Geometry check sheet. Reference: the model listing, model coordinates, mm. A direction names the side the tool comes from. Round coordinates to 2 decimals unless told otherwise and drop trailing zeros. Loops run counter-clockwise (first coordinate to the right, second up) from the corner with the lowest first, then second, coordinate; pieces in that order, holes last. Notation, with made-up numbers: M 35,-20 L 85,-20 A12 cw 85,-11 Z; hole C 63.25,41 d8. An arc over 180 degrees is marked long. Write item = value, one per line.
from build123d import *

# Parameters (mm, degrees)
F0_W     = 3
F0_H     = 30
F1_DEPTH = 52.5
F3_DEPTH = 25
F4_R     = 2
F6_DEPTH = 25


# Not quite as in the source:
# - a feature names something its author has since deleted; it is built from what else it names


with BuildPart() as f1:
    # F0 (on Top) → F1 (new body)
    with BuildSketch(Plane.XY):
        Polygon((2, 0), (-1, 0), (-6.1, 0), (-6.1, 30), (-9.1, 30), (-9.1, -2.9952730983), (40, -3), (40, 0), align=None)
        with Locations((0.5, 15)):
            Rectangle(F0_W, F0_H)
    extrude(amount=F1_DEPTH)

    # F2 (on face) → F3 (cut)
    with BuildSketch(Plane(origin=(-9.1, 0, 0), x_dir=(0, -1, 0), z_dir=(-1, 0, 0))):
        with BuildLine():
            Line((-13.5023634508, 37.5), (-13.5023634508, 39.25))
            ThreePointArc((-13.5023634508, 39.25), (-15.2523634508, 37.5), (-13.5023634508, 35.75))
            Line((-13.5023634508, 35.75), (-13.5023634508, 37.5))
        make_face()
        with BuildLine():
            ThreePointArc((-11.7523634508, 37.5), (-12.2649265837, 38.7374368671), (-13.5023634508, 39.25))
            Line((-13.5023634508, 39.25), (-13.5023634508, 37.5))
            Line((-13.5023634508, 37.5), (-13.5023634508, 35.75))
            ThreePointArc((-13.5023634508, 35.75), (-12.2649265837, 36.2625631329), (-11.7523634508, 37.5))
        make_face()
        with BuildLine():
            Line((-13.5023634508, 15), (-13.5023634508, 13.25))
            ThreePointArc((-13.5023634508, 13.25), (-12.2649265837, 13.7625631329), (-11.7523634508, 15))
            ThreePointArc((-11.7523634508, 15), (-12.2649265837, 16.2374368671), (-13.5023634508, 16.75))
            Line((-13.5023634508, 16.75), (-13.5023634508, 15))
        make_face()
        with BuildLine():
            ThreePointArc((-13.5023634508, 16.75), (-15.2523634508, 15), (-13.5023634508, 13.25))
            Line((-13.5023634508, 13.25), (-13.5023634508, 15))
            Line((-13.5023634508, 15), (-13.5023634508, 16.75))
        make_face()
    extrude(amount=-F3_DEPTH, mode=Mode.SUBTRACT)

    # F4
    f4_edges = [f1.edges().sort_by_distance(p)[0] for p in [
        (40, -1.5, 52.5),
        (-9.1, 30, 26.25),
        (-9.1, 13.502363, 52.5),
        (-7.6, 30, 52.5),
    ]]
    fillet(f4_edges, radius=F4_R)

    # F5 (on face) → F6 (cut)
    with BuildSketch(Plane(origin=(-0.000288442, -2.9961491359, 0), x_dir=(0.9999999954, -9.62709e-05, 0), z_dir=(-9.62709e-05, -0.9999999954, 0))):
        with BuildLine():
            Line((15.0002886274, 35), (15.0002886274, 33.25))
            ThreePointArc((15.0002886274, 33.25), (16.2377254944, 33.7625631329), (16.7502886274, 35))
            Line((16.7502886274, 35), (15.0002886274, 35))
        make_face()
        with BuildLine():
            ThreePointArc((15.0002886274, 36.75), (13.2502886274, 35), (15.0002886274, 33.25))
            Line((15.0002886274, 33.25), (15.0002886274, 35))
            Line((15.0002886274, 35), (15.0002886274, 36.75))
        make_face()
        with BuildLine():
            Line((15.0002886274, 36.75), (15.0002886274, 35))
            Line((15.0002886274, 35), (16.7502886274, 35))
            ThreePointArc((16.7502886274, 35), (16.2377254944, 36.2374368671), (15.0002886274, 36.75))
        make_face()
        with BuildLine():
            Line((30.0002886274, 35), (31.7502886274, 35))
            ThreePointArc((31.7502886274, 35), (31.2377254944, 36.2374368671), (30.0002886274, 36.75))
            Line((30.0002886274, 36.75), (30.0002886274, 35))
        make_face()
        with BuildLine():
            Line((28.2502886274, 35), (30.0002886274, 35))
            Line((30.0002886274, 35), (30.0002886274, 36.75))
            ThreePointArc((30.0002886274, 36.75), (28.7628517603, 36.2374368671), (28.2502886274, 35))
        make_face()
        with BuildLine():
            Line((30.0002886274, 33.25), (30.0002886274, 35))
            Line((30.0002886274, 35), (28.2502886274, 35))
            ThreePointArc((28.2502886274, 35), (28.7628517603, 33.7625631329), (30.0002886274, 33.25))
        make_face()
        with BuildLine():
            ThreePointArc((30.0002886274, 33.25), (31.2377254944, 33.7625631329), (31.7502886274, 35))
            Line((31.7502886274, 35), (30.0002886274, 35))
            Line((30.0002886274, 35), (30.0002886274, 33.25))
        make_face()
        with BuildLine():
            Line((30.0002886274, 15), (31.7502886274, 15))
            ThreePointArc((31.7502886274, 15), (31.2377254944, 16.2374368671), (30.0002886274, 16.75))
            Line((30.0002886274, 16.75), (30.0002886274, 15))
        make_face()
        with BuildLine():
            Line((28.2502886274, 15), (30.0002886274, 15))
            Line((30.0002886274, 15), (30.0002886274, 16.75))
            ThreePointArc((30.0002886274, 16.75), (28.7628517603, 16.2374368671), (28.2502886274, 15))
        make_face()
        with BuildLine():
            ThreePointArc((28.2502886274, 15), (28.7628517603, 13.7625631329), (30.0002886274, 13.25))
            Line((30.0002886274, 13.25), (30.0002886274, 15))
            Line((30.0002886274, 15), (28.2502886274, 15))
        make_face()
        with BuildLine():
            Line((30.0002886274, 15), (30.0002886274, 13.25))
            ThreePointArc((30.0002886274, 13.25), (31.2377254944, 13.7625631329), (31.7502886274, 15))
            Line((31.7502886274, 15), (30.0002886274, 15))
        make_face()
        with BuildLine():
            Line((15.0002886274, 15), (15.0002886274, 13.25))
            ThreePointArc((15.0002886274, 13.25), (16.2377254944, 13.7625631329), (16.7502886274, 15))
            Line((16.7502886274, 15), (15.0002886274, 15))
        make_face()
        with BuildLine():
            Line((15.0002886274, 16.75), (15.0002886274, 15))
            Line((15.0002886274, 15), (16.7502886274, 15))
            ThreePointArc((16.7502886274, 15), (16.2377254944, 16.2374368671), (15.0002886274, 16.75))
        make_face()
        with BuildLine():
            ThreePointArc((15.0002886274, 16.75), (13.2502886274, 15), (15.0002886274, 13.25))
            Line((15.0002886274, 13.25), (15.0002886274, 15))
            Line((15.0002886274, 15), (15.0002886274, 16.75))
        make_face()
    extrude(amount=-F6_DEPTH, mode=Mode.SUBTRACT)


solid = f1.part
(1) Material ranges on line 1 along X through (y, z) = (24, 7); line 2 along Y through (x, z) = (1.5, 33); line 3 along Y through (x, z) = (7, 50), recorded low to high. Write a range as from..to.
Result set:
line_1 = -9.1..-6.1, -1..2
line_2 = -3..30
line_3 = -3..0
(2) Depth check by flat-ended pin: pin 1 Ø2 at (x, z) = (3.5, 36.5) entering from +Y; pin 2 Ø4 at (x, z) = (10.5, 15.5) entering from -Y; pin 3 Ø6 at (y, z) = (25, 37) entering from +X; pin 4 Ø1.5 at (x, y) = (2, 18.5) entering from -Z. Enter the tip coordinate at first touch or a pass-through.
Result set:
pin_1 = 0
pin_2 = -3
pin_3 = 2
pin_4 = 0
(3) Release check for a two-part mould opening along X. For faces 1 (the flat face through (1, 9, 0)), 2 (the cylindrical face through (39.4, -1.48, 51.93)), 3 (the flat face through (-4, 0, 26)), 4 (the flat face through (-1, 15, 26)) record: released by +X, released by -X, zero draft, split by the parting line, or undercut.
Result set:
face_1 = zero draft
face_2 = released by +X
face_3 = undercut
face_4 = undercut
(4) Sectioned sample at B-B on z = 24.5. Record the cut outline in (x, y).
Result set:
outline = M -9.1,-3 L 40,-3 L 40,0 L 2,0 L 2,30 L -1,30 L -1,0 L -6.1,0 L -6.1,30 L -7.1,30 A2 ccw -9.1,28 Z
(5) Sectioned sample at A-A on y = 4.5. Record the cut outline in (x, z).
Result set:
outline = M -9.1,0 L -6.1,0 L -6.1,52.5 L -7.1,52.5 A2 ccw -9.1,50.5 Z; M -1,0 L 2,0 L 2,52.5 L -1,52.5 Z
(6) Tool access check on faces 5 (the cylindrical face through (-6.61, 29.4, 51.93)), 6 (the flat face through (40, -2, 25)), 7 (the flat face through (-6.1, 15, 26)), 8 (the flat face through (21, 0, 26)), 9 (the flat face through (0, 30, 26)). Record the directions out of +Z, -Z, +X, -X, +Y, -Y that give a thin tool (end or side, any length) a straight path to the whole face; none if there is none.
Result set:
face_5 = +Z, -X, +Y
face_6 = +Z, -Z, +X, +Y, -Y
face_7 = +Z, -Z, +Y
face_8 = +Z, -Z, +X, +Y
face_9 = +Z, -Z, +X, -X, +Y
(7) Sectioned sample at C-C on x = -2. Record the cut outline in (y, z), then the cut area to 3 significant figures.
Result set:
outline = M -3,0 L 0,0 L 0,52.5 L -3,52.5 Z
area = 157 mm2
